Design review of the part built by this model. Coordinates are the model's own, in mm. A direction names the side the tool comes from. Coordinates: 2 decimals unless noted, no trailing zeros. Write each loop counter-clockwise with the first axis right and the second up, starting at its lowest first coordinate (ties: lowest second). Pieces come first, ordered by that corner, then holes. Notation, with made-up numbers: (22.25, 89.5) - (28.25, 89.5) arc R27 cw to (28.25, 121.5) - close; hole circle Ø2 at (-26.75, -22). An arc over 180 degrees is marked (long way). Use a Markdown table: item, result.
from build123d import *
from build123d import SkipClean  # not in build123d's __all__

# Parameters (mm, degrees)
F0_R      = 8.5
F0_R_2    = 7
F1_DEPTH  = 150
F2_R      = 7
F2_R_2    = 5
F3_DEPTH  = 145
F4_W      = 30
F4_H      = 30
F4_R      = 8.5
F5_DEPTH  = 3
F7_D      = 4
F9_DEPTH  = 140
F12_ANGLE = 90
F14_DEPTH = 5
F15_W     = 2.5
F15_H     = 2.0939723571
F16_ANGLE = 90
F18_DEPTH = 10
F19_W     = 5
F19_H     = 2.0680303106
F20_ANGLE = 90
F22_DEPTH = 5
F23_W     = 5
F23_H     = 2.0939723571
F24_ANGLE = 90
F26_DEPTH = 10
F27_W     = 5
F27_H     = 2.0939723571
F28_ANGLE = 90
F30_DEPTH = 5


# Not quite as in the source:
# - after a boolean that leaves OpenCascade's solid faulty, fix() repairs it


with BuildPart() as f1:
    # F0 (on Right) → F1 (new body)
    with BuildSketch(Plane.YZ):
        Circle(F0_R)
        Circle(F0_R_2, mode=Mode.SUBTRACT)
    extrude(amount=F1_DEPTH)

    # F2 (on face) → F3 (join)
    with BuildSketch(Plane.YZ.offset(150)):
        Circle(F2_R)
        Circle(F2_R_2, mode=Mode.SUBTRACT)
    extrude(amount=-F3_DEPTH)

    # F4 (on face) → F5 (join)
    with BuildSketch(Plane(origin=(0, 0, 0), x_dir=(0, -1, 0), z_dir=(-1, 0, 0))):
        Rectangle(F4_W, F4_H)
        Circle(F4_R, mode=Mode.SUBTRACT)
    extrude(amount=-F5_DEPTH)

    # F7 (through all)
    with Locations(Plane(origin=(0, 0, 0), x_dir=(0, -1, 0), z_dir=(-1, 0, 0))):
        with Locations((-10, 10), (10, 10), (10, -10), (-10, -10)):
            Hole(F7_D / 2)

    # F8 (on face) → F9 (cut)
    with BuildSketch(Plane(origin=(5, 0, 0), x_dir=(0, -1, 0), z_dir=(-1, 0, 0))):
        with BuildLine():
            ThreePointArc((0, 5), (0.8891730726, 4.9203019467), (1.75, 4.6837484988))
            Line((1.75, 4.6837484988), (1.75, 6.7777208559))
            ThreePointArc((1.75, 6.7777208559), (0.8820300474, 6.9442078739), (0, 7))
            Line((0, 7), (0, 5))
        make_face()
        with BuildLine():
            ThreePointArc((-1.75, 4.6837484988), (-0.8891730726, 4.9203019467), (0, 5))
            Line((0, 5), (0, 7))
            ThreePointArc((0, 7), (-0.8820300474, 6.9442078739), (-1.75, 6.7777208559))
            Line((-1.75, 6.7777208559), (-1.75, 4.6837484988))
        make_face()
    extrude(amount=-F9_DEPTH, mode=Mode.SUBTRACT)

    # F10 (on face) → F12 (revolve, cut)
    with BuildSketch(Plane(origin=(0, -1.75, 0), x_dir=(-1, 0, 0), z_dir=(0, 1, 0))):
        Polygon((-140, 6.7777208559), (-140, 4.7096905453), (-140, 4.6837484988), (-135, 4.6837484988), (-135, 6.7777208559), align=None)
    revolve(axis=Axis((74.9857723713, 0, 0), (1, 0, 0)), revolution_arc=F12_ANGLE, mode=Mode.SUBTRACT)

    # F13 (on face) → F14 (cut)
    with BuildSketch(Plane(origin=(140, 0, 0), x_dir=(0, -1, 0), z_dir=(-1, 0, 0))):
        with BuildLine():
            Line((6.0300092452, 3.5551355111), (4.5493471919, 2.0744734578))
            ThreePointArc((4.5493471919, 2.0744734578), (4.9969153801, 0.17560377), (4.6837484988, -1.75))
            Line((4.6837484988, -1.75), (6.7777208559, -1.75))
            ThreePointArc((6.7777208559, -1.75), (6.9314935824, 0.9769322988), (6.0300092452, 3.5551355111))
        make_face()
    with SkipClean():  # cleaning this boolean's faces spoils the solid; the shape is the same uncleaned
        extrude(amount=-F14_DEPTH, mode=Mode.SUBTRACT)

    # F15 (on face) → F16 (revolve, cut)
    with BuildSketch(Plane(origin=(0, -1.75, 0), x_dir=(-1, 0, 0), z_dir=(0, 1, 0))):
        with Locations((-68.75, 5.7307346773)):
            Rectangle(F15_W, F15_H)
        with Locations((-71.25, 5.7307346773)):
            Rectangle(F15_W, F15_H)
    revolve(axis=Axis((74.9857723713, 0, 0), (1, 0, 0)), revolution_arc=F16_ANGLE, mode=Mode.SUBTRACT)

    add(f1.part.fix(), mode=Mode.REPLACE)

    # F17 (on face) → F18 (cut)
    with BuildSketch(Plane.YZ.offset(67.5)):
        with BuildLine():
            ThreePointArc((-4.6837484988, -1.75), (-4.9969153801, 0.17560377), (-4.5493471919, 2.0744734578))
            Line((-4.5493471919, 2.0744734578), (-6.0300092452, 3.5551355111))
            ThreePointArc((-6.0300092452, 3.5551355111), (-6.9314935824, 0.9769322988), (-6.7777208559, -1.75))
            Line((-6.7777208559, -1.75), (-4.6837484988, -1.75))
        make_face()
    extrude(amount=F18_DEPTH, mode=Mode.SUBTRACT)

    # F19 (on face) → F20 (revolve, cut)
    with BuildSketch(Plane(origin=(0, -1.75, 0), x_dir=(-1, 0, 0), z_dir=(0, 1, 0))):
        with Locations((-109.95097965, 5.8026228816)):
            Rectangle(F19_W, F19_H)
    revolve(axis=Axis((112.4786585569, 0, 0), (1, 0, 0)), revolution_arc=F20_ANGLE, mode=Mode.SUBTRACT)

    # F21 (on face) → F22 (cut)
    with BuildSketch(Plane(origin=(112.45097965, 0, 0), x_dir=(0, -1, 0), z_dir=(-1, 0, 0))):
        with BuildLine():
            ThreePointArc((6.8366380369, -1.75), (6.9854372426, 1.0028889159), (6.068155613, 3.6027221796))
            Line((6.068155613, 3.6027221796), (4.6366684016, 2.07447))
            ThreePointArc((4.6366684016, 2.07447), (5.0765586233, 0.1751347812), (4.7686077263, -1.75))
            Line((4.7686077263, -1.75), (6.8366380369, -1.75))
        make_face()
    extrude(amount=-F22_DEPTH, mode=Mode.SUBTRACT)

    # F23 (on face) → F24 (revolve, cut)
    with BuildSketch(Plane(origin=(0, -1.75, 0), x_dir=(-1, 0, 0), z_dir=(0, 1, 0))):
        with Locations((-33.75, 5.7307346773)):
            Rectangle(F23_W, F23_H)
    revolve(axis=Axis((74.9857723713, 0, 0), (1, 0, 0)), revolution_arc=F24_ANGLE, mode=Mode.SUBTRACT)

    # F25 (on face) → F26 (cut)
    with BuildSketch(Plane.YZ.offset(31.25)):
        with BuildLine():
            ThreePointArc((-4.6837484988, -1.75), (-4.9969153801, 0.17560377), (-4.5493471919, 2.0744734578))
            Line((-4.5493471919, 2.0744734578), (-6.0300092452, 3.5551355111))
            ThreePointArc((-6.0300092452, 3.5551355111), (-6.9314935824, 0.9769322988), (-6.7777208559, -1.75))
            Line((-6.7777208559, -1.75), (-4.6837484988, -1.75))
        make_face()
    extrude(amount=F26_DEPTH, mode=Mode.SUBTRACT)

    # F27 (on face) → F28 (revolve)
    with BuildSketch(Plane(origin=(0, -1.75, 0), x_dir=(-1, 0, 0), z_dir=(0, 1, 0))):
        with Locations((-7.5, 5.7307346773)):
            Rectangle(F27_W, F27_H)
    revolve(axis=Axis((74.9857723713, 0, 0), (1, 0, 0)), revolution_arc=F28_ANGLE)

    # F29 (on face) → F30 (cut)
    with BuildSketch(Plane(origin=(5, 0, 0), x_dir=(0, -1, 0), z_dir=(-1, 0, 0))):
        with BuildLine():
            Line((5.896972825, 3.7716987554), (4.4710360492, 2.2382664379))
            ThreePointArc((4.4710360492, 2.2382664379), (4.9875229666, 0.3530080143), (4.7417252408, -1.5862035621))
            Line((4.7417252408, -1.5862035621), (6.8179145096, -1.5862035621))
            ThreePointArc((6.8179145096, -1.5862035621), (6.8988310092, 1.185803823), (5.896972825, 3.7716987554))
        make_face()
    extrude(amount=-F30_DEPTH, mode=Mode.SUBTRACT)

    add(f1.part.fix(), mode=Mode.REPLACE)


solid = f1.part
(1) Machinability: for faces 4 (the cylindrical face through (2, -10, 12)), 5 (the flat face through (41.25, -6, 1)), 6 (the flat face through (5, 4, -4)), which of the approach directions +Z, -Z, +X, -X, +Y, -Y give a long, thin tool a straight path to every point of the face, cutting with its end or side? Answer none if there is none.
Determined:
| item | result |
|---|---|
| face 4 | +X, -X |
| face 5 | none |
| face 6 | -X |
(2) Draft analysis for pull direction Z (two halves, no side actions). For faces 1 (the flat face through (150, 4, -4)), 2 (the cylindrical face through (75.471, 4.57, 7.167)), 3 (the flat face through (67.5, -5, 3)), state which applies: +Z half, -Z half, draft (parallel to the pull), parting line (faces both ways), or undercut.
Determined:
| item | result |
|---|---|
| face 1 | draft |
| face 2 | parting line |
| face 3 | undercut |
(3) Take a section at A-A on y = 10. Write out the cut boundary in (x, z), and give its area (3 significant figures).
Determined:
| item | result |
|---|---|
| outline | (0, -15) - (3, -15) - (3, -12) - (0, -12) - close; (0, -8) - (3, -8) - (3, 8) - (0, 8) - close; (0, 12) - (3, 12) - (3, 15) - (0, 15) - close |
| area | 66.0 mm2 |
(4) Take a section at C-C on x = 120. Write out the cut boundary in (y, z).
Determined:
| item | result |
|---|---|
| outline | circle Ø17 at (0, 0); hole (-1.75, 4.68) arc R5 ccw (long way) to (1.75, 4.68) - (1.75, 6.78) arc R7 ccw to (-1.75, 6.78) - close |
(5) For pin 1 (0.6 mm diameter, centred on x = 140.5, y = -6, fed in from +Z); pin 2 (3 mm diameter, centred on y = 10, z = -10, fed in from -X); pin 3 (1 mm diameter, centred on x = 25, z = -4.5, fed in from +Y); pin 4 (10 mm diameter, centred on x = 55.5, y = 1.5, fed in from +Z), all flat-tipped, find the tip position at first contact; note any pin that passes through.
Determined:
| item | result |
|---|---|
| pin 1 | z = 6.31 |
| pin 2 | through |
| pin 3 | y = 7.5 |
| pin 4 | z = 8.5 |
(6) For L1, parallel to Z at x = 1.5, y = -10; L2, parallel to Y at x = 1.5, z = 0; L3, parallel to Y at x = 3.75, z = 0, list the stretches that pass through material, from the lowest coordinate up. Write a range as from..to.
Determined:
| item | result |
|---|---|
| L1 | -15..-12, -8..8, 12..15 |
| L2 | -15..-7, 7..15 |
| L3 | -8.5..-7, 7..8.5 |
(7) Take a section at D-D on z = 0. State how many separate pieces and enclosed holes the cut face has, and give its area (3 significant figures).
Determined:
| item | result |
|---|---|
| separate pieces | 2 |
| enclosed holes | 1 |
| area | 979 mm2 |
